Verification items for the finished model (mm, model axes). Give positions to 0.01 mm unless a question says otherwise; leave off trailing zeros. Loops run counter-clockwise (first coordinate to the right, second up) from the corner with the lowest first, then second, coordinate; pieces in that order, holes last. Notation, with made-up numbers: (49.25, -32.5) - (98.25, -32.5) arc R14 cw to (98.25, -26.5) - close; hole circle Ø9 at (-17.5, 82). An arc over 180 degrees is marked (long way). One line per item, written item: value. Start each with the question number.
1. Sectioned sample at B-B (x = 1.5). Record the cut outline in (y, z).
2. Sectioned sample at D-D (x = -2.25). Record the cut outline in (y, z), plus the area to 3 significant figures.
3. Sectioned sample at A-A (z = 0). Record the cut outline in (x, y).
4. Scan lines: L1, parallel to X at y = 0.1, z = 0; L2, parallel to X at y = 0.1, z = 1; L3, parallel to Z at x = 1.75, y = 0.2. Record each from-to range of solid material in increasing order. Write a range as [from, to].
5. Mould release check, pull along X, two halves, no side actions. Record for faces 1 (the flat face through (-3.4, 0, -0.1)), 2 (the cylindrical face through (0.9, 0.16, 2.86)), 3 (the cylindrical face through (-7.81, 0.16, -1.73)): pulls with the +X half, pulls with the -X half, needs draft (parallel to the pull), parting line crosses it, or undercut.
6. Sectioned sample at C-C (y = 0.2). Record the cut outline in (x, z), plus the area to 3 significant figures.
7. Gauge pin test, flat end, axial feed: pin 1 (1.5 mm diameter, centred on x = 4, z = -1.5, fed in from -Y). Record the tip position at first contact, or that the pin passes through.
from build123d import *

# Parameters (mm, degrees)
SKETCH1_R           = 7
BOSS_EXTRUDE1_DEPTH = 0.3175
SKETCH2_R           = 8
BOSS_EXTRUDE3_DEPTH = 0.3175
SKETCH3_R           = 1.5
CUT_EXTRUDE2_DEPTH  = 0.3175
SKETCH4_R           = 1.5
CUT_EXTRUDE3_DEPTH  = 0.3175
SKETCH5_R           = 3
CUT_EXTRUDE4_DEPTH  = 0.3175


with BuildPart() as part:
    # Sketch1 → Boss-Extrude1 (new body)
    with BuildSketch(Plane(origin=(0, 0, 0), x_dir=(1, 0, 0), z_dir=(0, 1, 0))):
        with Locations(Location((0, 0, 0), (0, 0, 270))):
            Circle(SKETCH1_R)
    extrude(amount=BOSS_EXTRUDE1_DEPTH)

    # Sketch2 → Boss-Extrude3 (add)
    with BuildSketch(Plane(origin=(0, 0.3175, 0), x_dir=(1, 0, 0), z_dir=(0, 1, 0))):
        with Locations(Location((0, 0, 0), (0, 0, 270))):
            Circle(SKETCH2_R)
    extrude(amount=-BOSS_EXTRUDE3_DEPTH)

    # Sketch3 → Cut-Extrude2 (cut)
    with BuildSketch(Plane(origin=(0, 0.3175, 0), x_dir=(1, 0, 0), z_dir=(0, 1, 0))):
        with Locations(Location((6, 0, 0), (0, 0, 270))):
            Circle(SKETCH3_R)
    extrude(amount=-CUT_EXTRUDE2_DEPTH, mode=Mode.SUBTRACT)

    # Sketch4 → Cut-Extrude3 (cut)
    with BuildSketch(Plane(origin=(0, 0.3175, 0), x_dir=(1, 0, 0), z_dir=(0, 1, 0))):
        with Locations(Location((-6, 0, 0), (0, 0, 270))):
            Circle(SKETCH4_R)
    extrude(amount=-CUT_EXTRUDE3_DEPTH, mode=Mode.SUBTRACT)

    # Sketch5 → Cut-Extrude4 (cut)
    with BuildSketch(Plane(origin=(0, 0.3175, 0), x_dir=(1, 0, 0), z_dir=(0, 1, 0))):
        with Locations(Location((0, 0, 0), (0, 0, 270))):
            Circle(SKETCH5_R)
    extrude(amount=-CUT_EXTRUDE4_DEPTH, mode=Mode.SUBTRACT)


solid = part.part
Results are:
1. outline: (0, -7.86) - (0.32, -7.86) - (0.32, -2.6) - (0, -2.6) - close; (0, 2.6) - (0.32, 2.6) - (0.32, 7.86) - (0, 7.86) - close
2. outline: (0, -7.68) - (0.32, -7.68) - (0.32, -1.98) - (0, -1.98) - close; (0, 1.98) - (0.32, 1.98) - (0.32, 7.68) - (0, 7.68) - close
2. area: 3.61 mm^2
3. outline: (-8, 0) - (-7.5, 0) - (-7.5, 0.32) - (-8, 0.32) - close; (-4.5, 0) - (-3, 0) - (-3, 0.32) - (-4.5, 0.32) - close; (3, 0) - (4.5, 0) - (4.5, 0.32) - (3, 0.32) - close; (7.5, 0) - (8, 0) - (8, 0.32) - (7.5, 0.32) - close
4. L1: x = [-8, -7.5], [-4.5, -3], [3, 4.5], [7.5, 8]
4. L2: x = [-7.94, -7.12], [-4.88, -2.83], [2.83, 4.88], [7.12, 7.94]
4. L3: z = [-7.81, -2.44], [2.44, 7.81]
5. face 1: needs draft
5. face 2: undercut
5. face 3: parting line crosses it
6. outline: circle Ø16 at (0, 0); hole circle Ø3 at (-6, 0); hole circle Ø6 at (0, 0); hole circle Ø3 at (6, 0)
6. area: 159 mm^2
7. pin 1: stops at y = 0
